Check sheet for the drawn part. Datum: minimum x, y, z corner. Units: mm. A direction names the side the tool comes from. Give positions to 0.01 mm unless a question says otherwise; leave off trailing zeros. Loops run counter-clockwise (first coordinate to the right, second up) from the corner with the lowest first, then second, coordinate; pieces in that order, holes last.
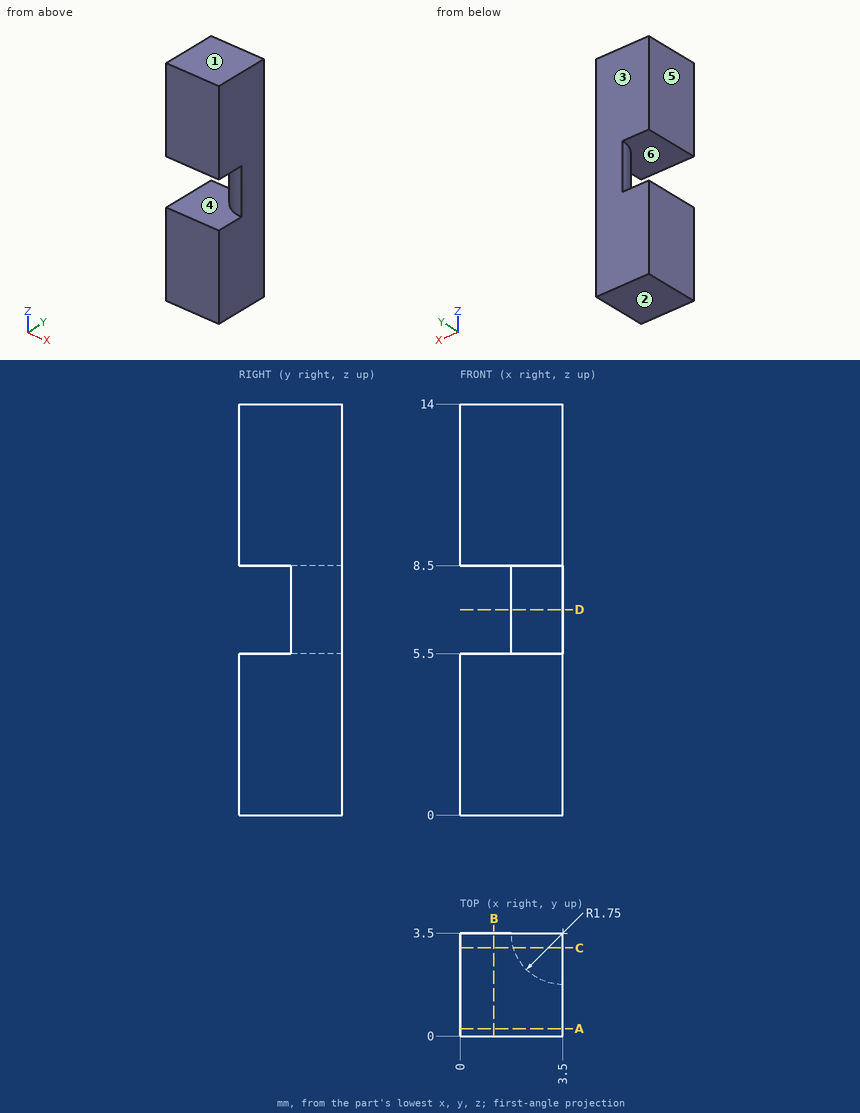
1) Sectioned sample at D-D on z = 7. Enter the section's corners in (x, y), plus the area to 3 significant figures.
2) Scan lines: line 1 along Z through (x, y) = (0.4, 1.25); line 2 along X through (y, z) = (2.95, 6); line 3 along Y through (x, z) = (2.55, 5.75). Record each from-to range of solid material in increasing order.
3) Mould release check, pull along Z, two halves, no side actions. Record for the marked faces 1, 2, 3 and 4: +Z half, -Z half, draft (parallel to the pull), parting line (faces both ways), or undercut.
4) Sectioned sample at C-C on y = 3. Enter the section's corners in (x, z).
5) Sectioned sample at A-A on y = 0.25. Enter the section's corners in (x, z), plus the area to 3 significant figures.
6) Tool access check on the marked faces 5 and 6. Record the directions out of +Z, -Z, +X, -X, +Y, -Y that give a thin tool (end or side, any length) a straight path to the whole face; none if there is none.
Determined:
1. outline: (1.75, 3.5) arc R1.75 ccw to (3.5, 1.75) - (3.5, 3.5) - close
1. area: 2.41 mm2
2. line 1: z = 0 to 5.5, 8.5 to 14
2. line 2: x = 1.84 to 3.5
2. line 3: y = 2.03 to 3.5
3. face 1: +Z half
3. face 2: -Z half
3. face 3: draft
3. face 4: undercut
4. outline: (0, 0) - (3.5, 0) - (3.5, 14) - (0, 14) - (0, 8.5) - (1.82, 8.5) - (1.82, 5.5) - (0, 5.5) - close
5. outline: (0, 0) - (3.5, 0) - (3.5, 5.5) - (0, 5.5) - close; (0, 8.5) - (3.5, 8.5) - (3.5, 14) - (0, 14) - close
5. area: 38.5 mm2
6. face 5: +Z, -Z, -X, +Y, -Y
6. face 6: -X, -Y
